```python
from build123d import *

# Parameters (mm, degrees)
SKETCH_1_R           = 1.7
SKETCH_1_R_2         = 1
EXTRUDE_1_DEPTH      = 0.9
EXTRUDE_1_DEPTH_BACK = 2
SKETCH_1_3_R         = 5.7
SKETCH_1_3_R_2       = 4.525
EXTRUDE_2_DEPTH      = 1.5
SKETCH_2_R           = 5
EXTRUDE_3_DEPTH      = 1.2
SKETCH_2_5_R         = 1
CUT_EXTRUDE_3_DEPTH  = 2.2
SKETCH_6_R           = 1.15
CUT_EXTRUDE_4_DEPTH  = 0.9
SKETCH_4_W           = 0.5
SKETCH_4_H           = 0.375
SKETCH_7_R           = 5.325
CUT_EXTRUDE_5_DEPTH  = 0.7


with BuildPart() as part:
    # Sketch 1 → Extrude 1 (new body, two sides)
    with BuildSketch(Plane.XY) as extrude_1_sk:
        Circle(SKETCH_1_R)
        Circle(SKETCH_1_R_2, mode=Mode.SUBTRACT)
    extrude(amount=EXTRUDE_1_DEPTH)
    extrude(extrude_1_sk.sketch, amount=-EXTRUDE_1_DEPTH_BACK)

    # Sketch 2 → Extrude 3 (add)
    with BuildSketch(Plane(origin=(0, 0, -2), x_dir=(-1, 0, 0), z_dir=(0, 0, -1))):
        Circle(SKETCH_2_R)
    extrude(amount=EXTRUDE_3_DEPTH)

    # Sketch 2_5 → Cut-Extrude 3 (cut, through all)
    with BuildSketch(Plane(origin=(0, 0, -2), x_dir=(-1, 0, 0), z_dir=(0, 0, -1))):
        with BuildLine():
            Line((-0.7, -1.549193338), (-0.7, -2.19089023))
            ThreePointArc((-0.7, -2.19089023), (0, -2.3), (0.7, -2.19089023))
            Line((0.7, -2.19089023), (0.7, -1.549193338))
            ThreePointArc((0.7, -1.549193338), (0, -1.7), (-0.7, -1.549193338))
        make_face()
        with BuildLine():
            ThreePointArc((0.7, 2.19089023), (0, 2.3), (-0.7, 2.19089023))
            Line((-0.7, 2.19089023), (-0.7, 1.549193338))
            ThreePointArc((-0.7, 1.549193338), (0, 1.7), (0.7, 1.549193338))
            Line((0.7, 1.549193338), (0.7, 2.19089023))
        make_face()
        with BuildLine():
            Line((-0.7, -1.549193338), (-0.7, -2.19089023))
            ThreePointArc((-0.7, -2.19089023), (0, -2.3), (0.7, -2.19089023))
            Line((0.7, -2.19089023), (0.7, -1.549193338))
            ThreePointArc((0.7, -1.549193338), (0, -1.7), (-0.7, -1.549193338))
        make_face()
        with BuildLine():
            ThreePointArc((0.7, 2.19089023), (0, 2.3), (-0.7, 2.19089023))
            Line((-0.7, 2.19089023), (-0.7, 1.549193338))
            ThreePointArc((-0.7, 1.549193338), (0, 1.7), (0.7, 1.549193338))
            Line((0.7, 1.549193338), (0.7, 2.19089023))
        make_face()
        with Locations(Location((0, 0, 0), (0, 0, 180))):  # turned: the seam where the file's is
            Circle(SKETCH_2_5_R)
    extrude(amount=CUT_EXTRUDE_3_DEPTH, mode=Mode.SUBTRACT)

    # Sketch 6 → Cut-Extrude 4 (cut)
    with BuildSketch(Plane(origin=(0, 0, -3.2), x_dir=(-1, 0, 0), z_dir=(0, 0, -1))):
        Circle(SKETCH_6_R)
    extrude(amount=-CUT_EXTRUDE_4_DEPTH, mode=Mode.SUBTRACT)



with BuildPart() as body_2:
    # Sketch 1_3 → Extrude 2 (new body)
    with BuildSketch(Plane.XY):
        Circle(SKETCH_1_3_R)
        Circle(SKETCH_1_3_R_2, mode=Mode.SUBTRACT)
    extrude(amount=-EXTRUDE_2_DEPTH)


with BuildPart() as part_1:
    add(part.part)

    add(body_2.part)  # Revolve 2 merges body 2
    # Sketch 4 → Revolve 2 (revolve)
    with BuildSketch(Plane(origin=(0, 0, 0), x_dir=(0, 0, -1), z_dir=(1, 0, 0)), mode=Mode.PRIVATE) as revolve_2_sk:
        Polygon((1.5, 5.7), (5.5, 6.2), (5.5, 4.9), (1.5, 4.9), align=None)
        with Locations((1.75, 4.7125)):
            Rectangle(SKETCH_4_W, SKETCH_4_H)
    revolve(revolve_2_sk.sketch.rotate(Axis((0, 0, 1000), (0, 0, -1)), 90), axis=Axis((0, 0, 1000), (0, 0, -1)))  # turned: the seam where the file's is

    # Sketch 7 → Cut-Extrude 5 (cut)
    with BuildSketch(Plane(origin=(0, 0, -5.5), x_dir=(-1, 0, 0), z_dir=(0, 0, -1))):
        Circle(SKETCH_7_R)
    extrude(amount=-CUT_EXTRUDE_5_DEPTH, mode=Mode.SUBTRACT)


solid = part_1.part
```
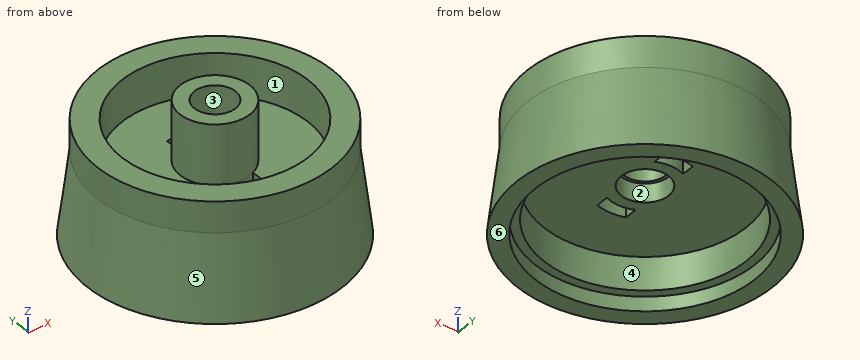
Work out the finished part from the listing and answer in its coordinate system (mm). Face numbers are marked on the shaded views. A direction names the side the tool comes from. Round coordinates to 2 decimals unless told otherwise and drop trailing zeros. Write each loop counter-clockwise with the first axis right and the second up, starting at its lowest first coordinate (ties: lowest second). Pieces come first, ordered by that corner, then holes. Notation, with made-up numbers: (29, -11) -> (50, -11) arc R21 ccw to (50, 22) -> close; hole circle Ø8 at (-6, 82.25). An arc over 180 degrees is marked (long way). Write each question's results on one line, items separated by ' | '.
Q1. Determine the mould class of the marked faces 4, 5 and 6 for opening direction Y: released by +Y, released by -Y, zero draft, split by the parting line, or undercut.
Data:
face 4: undercut | face 5: split by the parting line | face 6: zero draft
Q2. Flat-ended cylindrical pins translate along their axes: P1, Ø2, axis at y = -1.5, z = -3.5, coming from the +X side; P2, Ø1.6, axis at x = 0, y = 0, coming from the +Z side; P3, Ø7, axis at x = 0, y = 0, coming from the -Z side; P4, Ø6, axis at x = -0.5, y = -2.5, coming from the -Z side. Find the tip coordinate at first contact, or state that the pin passes through.
Data:
P1: x = 5.99 | P2: through | P3: z = -3.2 | P4: z = -5.5
Q3. Straight lines are drawn through the part: line 1 along Y through (x, z) = (0, -1) (3 decimals); line 2 along Y through (x, z) = (0, 0.75); line 3 along Z through (x, y) = (1.5, 0.5). For each, find the intervals that lie inside material, in ascending order. Write a range as [from, to].
Data:
line 1: [-5.7, -4.525], [-1.7, -1], [1, 1.7], [4.525, 5.7] | line 2: [-1.7, -1], [1, 1.7] | line 3: [-3.2, 0.9]
Q4. Section B-B, the plane x = 0 is taken. Give the number of separate pieces and of enclosed holes in the cut face, then the cut area to 3 significant figures.
Data:
separate pieces: 4 | enclosed holes: 0 | area: 23.4 mm^2
Q5. Which of the six approach directions +Z, -Z, +X, -X, +Y, -Y give full straight-line access (tool end or side, diameter ignored) to the marked faces 1, 2 and 3?
Data:
face 1: +Z | face 2: -Z | face 3: +Z, -Z
Q6. Section C-C, the plane z = -3.5 is taken. Write down the section's boundary in (x, y).
Data:
outline: circle Ø11.9 at (0, 0); hole circle Ø9.8 at (0, 0)
